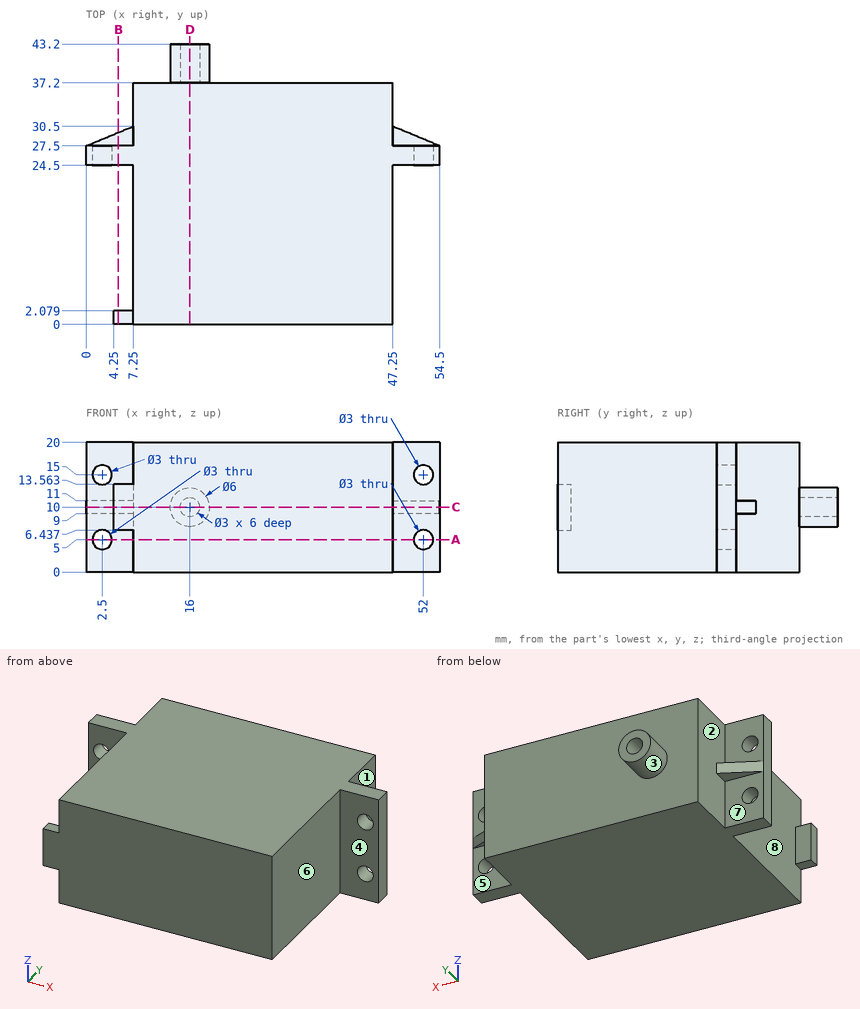
Study the drawing (mm; zero at the part's minimum x, y, z) and answer. A direction names the side the tool comes from. Round coordinates to 2 decimals unless told otherwise and drop trailing zeros. Write each loop counter-clockwise with the first axis right and the second up, starting at its lowest first coordinate (ties: lowest second). Pieces come first, ordered by that corner, then holes.
1) A cutting plane is placed at B-B (x = 5). Give the vertices of the cut face in (y, z).
2) A cutting plane is placed at A-A (z = 5). Give the vertices of the cut face in (x, y).
3) A tool of negligible diameter and unlimited length cuts with its end or side. For the marked faces 1, 2, 3, 4 and 5, from which of +Z, -Z, +X, -X, +Y, -Y can it reach the whole face along a straight path? Write none if from no direction.
4) A cutting plane is placed at C-C (z = 10). Give the vertices of the cut face in (x, y).
5) Straight lines are drawn through the part: line 1 (X direction, y = 26.7, z = 15); line 2 (X direction, y = 41.95, z = 10); line 3 (Z direction, x = 2, y = 25) (1 decimal). For each, find the intervals that lie inside material, in ascending order.
6) The mould has two halves that part along Y. Classify the marked faces 6, 7 and 8: pulls with the +Y half, pulls with the -Y half, needs draft (parallel to the pull), parting line crosses it, or undercut.
7) A cutting plane is placed at D-D (x = 16). Give the vertices of the cut face in (y, z), plus the area to 3 significant figures.
8) Given pin 1 Ø10 at (y, z) = (13.5, 7.5) entering from -X; pin 2 Ø10 at (x, y) = (20, 35.5) entering from -Z; pin 3 Ø8 at (x, z) = (5, 6) entering from +Y; pin 4 Ø1 at (x, y) = (6, 1) entering from +Z, each flat-ended and moving along its own axis, determine where each tip first touches the part or whether it passes through.
Completed:
1. outline: (0, 6.44) - (2.08, 6.44) - (2.08, 13.56) - (0, 13.56) - close; (24.5, 0) - (27.5, 0) - (27.5, 9) - (29.57, 9) - (29.57, 11) - (27.5, 11) - (27.5, 20) - (24.5, 20) - close
2. outline: (0, 24.5) - (1, 24.5) - (1, 27.5) - (0, 27.5) - close; (4, 24.5) - (7.25, 24.5) - (7.25, 0) - (47.25, 0) - (47.25, 24.5) - (50.5, 24.5) - (50.5, 27.5) - (47.25, 27.5) - (47.25, 37.2) - (7.25, 37.2) - (7.25, 27.5) - (4, 27.5) - close; (53.5, 24.5) - (54.5, 24.5) - (54.5, 27.5) - (53.5, 27.5) - close
3. face 1: +X, +Y
3. face 2: -X, +Y
3. face 3: +Y
3. face 4: +Z, -Z, +X, -Y
3. face 5: -Z, +X, +Y
4. outline: (0, 24.5) - (7.25, 24.5) - (7.25, 2.08) - (4.25, 2.08) - (4.25, 0) - (47.25, 0) - (47.25, 24.5) - (54.5, 24.5) - (54.5, 27.5) - (47.25, 30.5) - (47.25, 37.2) - (19, 37.2) - (19, 43.2) - (17.5, 43.2) - (17.5, 37.2) - (14.5, 37.2) - (14.5, 43.2) - (13, 43.2) - (13, 37.2) - (7.25, 37.2) - (7.25, 30.5) - (0, 27.5) - close
5. line 1: x = 0 to 1, 4 to 50.5, 53.5 to 54.5
5. line 2: x = 13 to 14.5, 17.5 to 19
5. line 3: z = 0 to 3.6, 6.4 to 13.6, 16.4 to 20
6. face 6: needs draft
6. face 7: pulls with the +Y half
6. face 8: undercut
7. outline: (0, 0) - (37.2, 0) - (37.2, 7) - (43.2, 7) - (43.2, 8.5) - (37.2, 8.5) - (37.2, 11.5) - (43.2, 11.5) - (43.2, 13) - (37.2, 13) - (37.2, 20) - (0, 20) - close
7. area: 762 mm2
8. pin 1: stops at x = 7.25
8. pin 2: stops at z = 0
8. pin 3: stops at y = 37.2
8. pin 4: stops at z = 13.56
